Build history of the part. All positions in model axes, mm. Give positions to 0.01 mm unless a question says otherwise; leave off trailing zeros. Order: outer loops, then holes, each group sorted by start corner. A loop starts at its lowest first (then second) coordinate and runs counter-clockwise, first axis right, second up. Notation, with made-up numbers: M 13.5,41 L 31.5,41 A21 ccw 31.5,52 Z; hole C 22.25,-0.5 d5. An arc over 180 degrees is marked long. Answer as CSV lines item,"result".
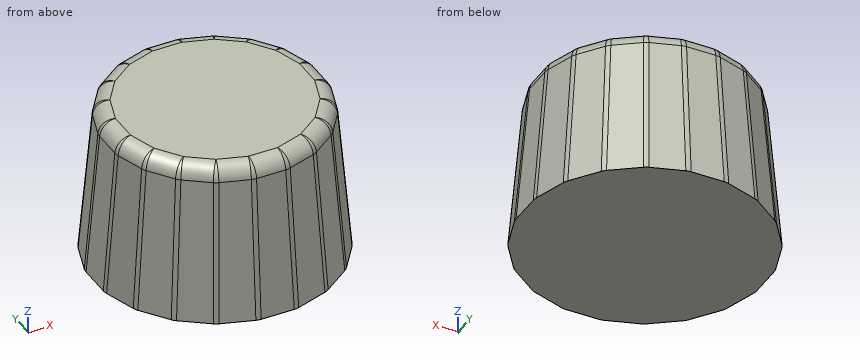
from build123d import *

# Parameters (mm, degrees)
F1_DEPTH = 20
F1_TAPER = 5
F2_R     = 2


with BuildPart() as f1:
    # F0 (on Top) → F1 (new body)
    with BuildSketch(Plane.XY):
        Polygon((15.2196083218, -2.410549146), (15.2196083218, 2.410549146), (13.729807018, 6.9956860923), (10.8960365421, 10.8960365421), (6.9956860923, 13.729807018), (2.410549146, 15.2196083218), (-2.410549146, 15.2196083218), (-6.9956860923, 13.729807018), (-10.8960365421, 10.8960365421), (-13.729807018, 6.9956860923), (-15.2196083218, 2.410549146), (-15.2196083218, -2.410549146), (-13.729807018, -6.9956860923), (-10.8960365421, -10.8960365421), (-6.9956860923, -13.729807018), (-2.410549146, -15.2196083218), (2.410549146, -15.2196083218), (6.9956860923, -13.729807018), (10.8960365421, -10.8960365421), (13.729807018, -6.9956860923), align=None)
    extrude(amount=F1_DEPTH, taper=F1_TAPER)

    # F2
    f2_edges = [f1.edges().sort_by_distance(p)[0] for p in [
        (0, 13.469835, 20),
        (4.162408, 12.810574, 20),
        (7.91737, 10.897325, 20),
        (-10.897325, 7.91737, 20),
        (-12.810574, -4.162408, 20),
        (-10.897325, -7.91737, 20),
        (-7.91737, -10.897325, 20),
        (-4.162408, -12.810574, 20),
        (0, -13.469835, 20),
        (4.162408, -12.810574, 20),
        (7.91737, -10.897325, 20),
        (10.897325, -7.91737, 20),
        (12.810574, -4.162408, 20),
        (13.469835, 0, 20),
        (12.810574, 4.162408, 20),
        (10.897325, 7.91737, 20),
        (-4.162408, 12.810574, 20),
        (-7.91737, 10.897325, 20),
        (-12.810574, 4.162408, 20),
        (-13.469835, 0, 20),
        (2.271981, 14.344722, 10),
        (-2.271981, 14.344722, 10),
        (-6.593545, 12.94056, 10),
        (-10.269687, 10.269687, 10),
        (-12.94056, 6.593545, 10),
        (-14.344722, 2.271981, 10),
        (-14.344722, -2.271981, 10),
        (-12.94056, -6.593545, 10),
        (-10.269687, -10.269687, 10),
        (-6.593545, -12.94056, 10),
        (-2.271981, -14.344722, 10),
        (2.271981, -14.344722, 10),
        (6.593545, -12.94056, 10),
        (10.269687, -10.269687, 10),
        (12.94056, 6.593545, 10),
        (6.593545, 12.94056, 10),
        (10.269687, 10.269687, 10),
        (14.344722, 2.271981, 10),
        (14.344722, -2.271981, 10),
        (12.94056, -6.593545, 10),
    ]]
    fillet(f2_edges, radius=F2_R)


solid = f1.part
Item 1: Band-saw the part on A-A (x = 1). Give the cut face in (y, z).
Geometry says:
outline,"M -15.22,0 L 15.22,0 L 13.63,18.17 A2 ccw 11.64,20 L -11.64,20 A2 ccw -13.63,18.17 Z"
Item 2: Drop flat-ended pins along their axis: pin 1 (1.5 mm diameter, centred on y = 0, z = 6, fed in from -X); pin 2 (1 mm diameter, centred on y = 11.5, z = 5, fed in from -X); pin 3 (6 mm diameter, centred on y = -9, z = 4, fed in from +X). Give the stop position or say it passes through.
Geometry says:
pin 1,"stops at x = -14.76"
pin 2,"stops at x = -10.01"
pin 3,"stops at x = 13.72"
Item 3: Probe line 1 along Y through (x, z) = (-7, 11.75); line 2 along Y through (x, z) = (-5.5, 2.25); line 3 along X through (y, z) = (-5.5, 14.25). List the from-to ranges inside material, lowest first. Write a range as from..to.
Geometry says:
line 1,"y = -12.46..12.46"
line 2,"y = -14.01..14.01"
line 3,"x = -12.9..12.9"
